Geometry: final body of the model. Coordinates: model frame, mm. Face numbers are marked on the shaded views. Coordinates: 2 decimals unless noted, no trailing zeros. Order: outer loops, then holes, each group sorted by start corner. A loop starts at its lowest first (then second) coordinate and runs counter-clockwise, first axis right, second up. Notation, with made-up numbers: M 86.5,-18 L 117.5,-18 A27 ccw 117.5,1 Z; hole C 3.25,-18 d3. An arc over 180 degrees is marked long. Use CSV: the item, a comma, the result in double quotes. Start each with the question number.
Q1. Mould query, pull axis Z, two halves, no side actions, for the marked faces 1 and 2. Classes: +Z half, -Z half, draft (parallel to the pull), parting line (faces both ways), or undercut.
Q2. Ray query, probe 1 along Y at (x, z) = (0, 0.85); probe 2 along X at (y, z) = (-25.5, 2.4); probe 3 along Y at (x, z) = (44, 1.25). Return the intervals inside material, ascending.
Q3. First-contact query: P1, Ø4, axis at x = 94.25, y = 25.25, coming from the -Z side; P2, Ø1.2, axis at y = -25, z = 2.5, coming from the -X side; P3, Ø6, axis at x = -94.5, y = -25.5, coming from the +Z side; P4, Ø3, axis at x = -94.25, y = 25.25, coming from the -Z side. Flat tips, straight axial feed; report the tip coordinate or a pass-through.
Q4. Section query D-D, the plane x = 94.25. Output: boundary loops of the cut face in (y, z), and give its area (3 significant figures).
Q5. Section query B-B, the plane z = 3.3. State how many separate pieces and enclosed holes the cut face has, and give its area (3 significant figures).
Q6. Section query A-A, the plane x = 0. Output: boundary loops of the cut face in (y, z), and give its area (3 significant figures).
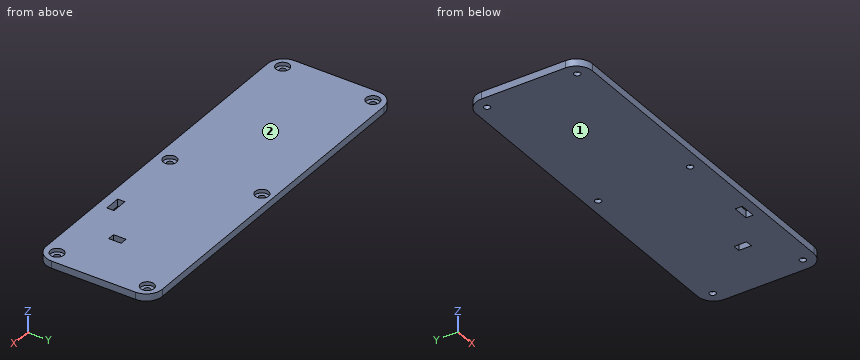
from build123d import *

# Parameters (mm, degrees)
F0_R     = 3.75
F0_W     = 9
F0_H     = 4
F0_W_2   = 4
F0_H_2   = 7
F1_DEPTH = 4
F0_R_2   = 1.75
F2_DEPTH = 2


with BuildPart() as f1:
    # F0 (on Top) → F1 (new body)
    with BuildSketch(Plane.XY):
        with BuildLine():
            Line((-92.5, -32.5), (92.5, -32.5))
            ThreePointArc((92.5, -32.5), (98.863961, -29.863961), (101.5, -23.5))
            Line((101.5, -23.5), (101.5, 23.5))
            ThreePointArc((101.5, 23.5), (98.863961, 29.863961), (92.5, 32.5))
            Line((92.5, 32.5), (-92.5, 32.5))
            ThreePointArc((-92.5, 32.5), (-98.863961, 29.863961), (-101.5, 23.5))
            Line((-101.5, 23.5), (-101.5, -23.5))
            ThreePointArc((-101.5, -23.5), (-98.863961, -29.863961), (-92.5, -32.5))
        make_face()
        with Locations((-94.25, -25.25)):
            Circle(F0_R, mode=Mode.SUBTRACT)
        with Locations((0, -25.25)):
            Circle(F0_R, mode=Mode.SUBTRACT)
        with Locations((45.54334, -25)):
            Rectangle(F0_W, F0_H, mode=Mode.SUBTRACT)
        with Locations((94.25, -25.25)):
            Circle(F0_R, mode=Mode.SUBTRACT)
        with Locations((68.991225, -8.446518)):
            Rectangle(F0_W_2, F0_H_2, mode=Mode.SUBTRACT)
        with Locations((-94.25, 25.25)):
            Circle(F0_R, mode=Mode.SUBTRACT)
        with Locations((0, 26.25)):
            Circle(F0_R, mode=Mode.SUBTRACT)
        with Locations((94.25, 25.25)):
            Circle(F0_R, mode=Mode.SUBTRACT)
    extrude(amount=F1_DEPTH)

    # F0 (on Top) → F2 (join)
    with BuildSketch(Plane.XY):
        with Locations((94.25, -25.25)):
            Circle(F0_R)
        with Locations((94.25, -25.25)):
            Circle(F0_R_2, mode=Mode.SUBTRACT)
        with Locations((0, -25.25)):
            Circle(F0_R)
        with Locations((0, -25.25)):
            Circle(F0_R_2, mode=Mode.SUBTRACT)
        with Locations((0, 26.25)):
            Circle(F0_R)
        with Locations((0, 26.25)):
            Circle(F0_R_2, mode=Mode.SUBTRACT)
        with Locations((94.25, 25.25)):
            Circle(F0_R)
        with Locations((94.25, 25.25)):
            Circle(F0_R_2, mode=Mode.SUBTRACT)
        with Locations((-94.25, -25.25)):
            Circle(F0_R)
        with Locations((-94.25, -25.25)):
            Circle(F0_R_2, mode=Mode.SUBTRACT)
        with Locations((-94.25, 25.25)):
            Circle(F0_R)
        with Locations((-94.25, 25.25)):
            Circle(F0_R_2, mode=Mode.SUBTRACT)
    extrude(amount=F2_DEPTH)


solid = f1.part
Responses:
1,face 1,"-Z half"
1,face 2,"+Z half"
2,probe 1,"y = -32.5 to -27, -23.5 to 24.5, 28 to 32.5"
2,probe 2,"x = -101.27 to -97.99, -90.51 to -3.74, 3.74 to 41.04, 50.04 to 90.51, 97.99 to 101.27"
2,probe 3,"y = -32.5 to -27, -23 to 32.5"
3,P1,"stops at z = 0"
3,P2,"stops at x = -101.45"
3,P3,"stops at z = 2"
3,P4,"passes through"
4,outline,"M -32.33,0 L -27,0 L -27,2 L -29,2 L -29,4 L -32.33,4 Z; M -23.5,0 L 23.5,0 L 23.5,2 L 21.5,2 L 21.5,4 L -21.5,4 L -21.5,2 L -23.5,2 Z; M 27,0 L 32.33,0 L 32.33,4 L 29,4 L 29,2 L 27,2 Z"
4,area,"215 mm²"
5,separate pieces,"1"
5,enclosed holes,"8"
5,area,"12,800 mm²"
6,outline,"M -32.5,0 L -27,0 L -27,2 L -29,2 L -29,4 L -32.5,4 Z; M -23.5,0 L 24.5,0 L 24.5,2 L 22.5,2 L 22.5,4 L -21.5,4 L -21.5,2 L -23.5,2 Z; M 28,0 L 32.5,0 L 32.5,4 L 30,4 L 30,2 L 28,2 Z"
6,area,"216 mm²"
